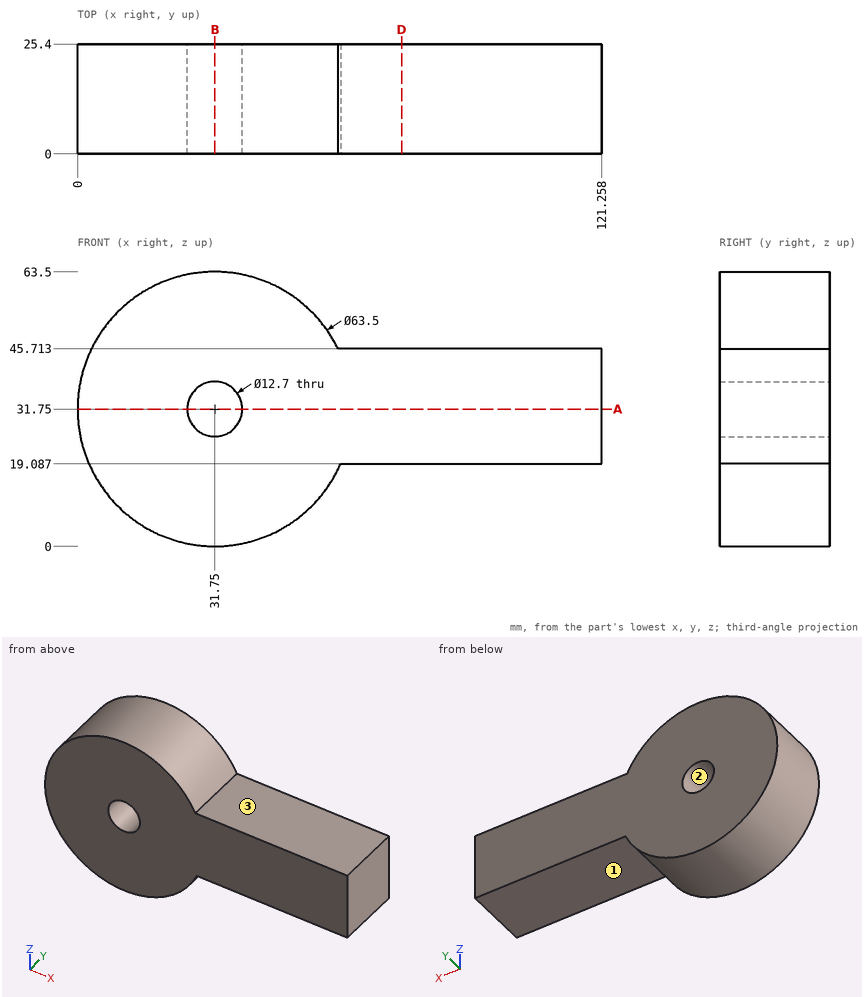
Could you check a few things on this drawing? It's one solid part, dimensions in mm from its lowest x, y, z. Coordinates: 2 decimals unless noted, no trailing zeros. Write each loop counter-clockwise with the first axis right and the second up, starting at its lowest first coordinate (ties: lowest second). Pieces come first, ordered by that corner, then holes. Notation, with made-up numbers: (46, 32) - (96, 32) arc R9 ccw to (96, 37) - close; hole circle Ø5 at (54.5, -36.5). An arc over 180 degrees is marked (long way). Put each result on its own line as item: value. Start each with the question number.
Q1. I want a section at A-A on z = 31.75. Write out the boundary of the cut face in (x, y), plus the area to 3 significant figures.
Q2. Please list where these lines run through material, in increasing order: L1, parallel to Z at x = 31.75, y = 14.5; L2, parallel to X at y = 20, z = 31.75; L3, parallel to Z at x = 112.5, y = 20.
Q3. I want a section at D-D on x = 75. Write out the boundary of the cut face in (y, z).
Q4. Thinking about a two-plate mould opening in Z: for the marked faces 1, 2 and 3, which applies, pulls with the +Z half, pulls with the -Z half, needs draft (parallel to the pull), parting line crosses it, or undercut?
Q5. I'm going to push flat-ended pins straight in: P1, Ø1, axis at y = 6.5, z = 15.5, coming from the +X side; P2, Ø1, axis at x = 35.5, y = 10, coming from the -Z side; P3, Ø5, axis at y = 3, z = 27.5, coming from the -X side; P4, Ø14.5, axis at x = 31.75, z = 31.75, coming from the -Y side. Where does each tip first touch, or does it pass through?
Q6. I want a section at B-B on x = 31.75. Write out the boundary of the cut face in (y, z).
Checks:
1. outline: (0, 0) - (25.4, 0) - (25.4, 25.4) - (0, 25.4) - close; (38.1, 0) - (121.26, 0) - (121.26, 25.4) - (38.1, 25.4) - close
1. area: 2,760 mm²
2. L1: 0 to 25.4, 38.1 to 63.5
2. L2: 0 to 25.4, 38.1 to 121.26
2. L3: 19.09 to 45.71
3. outline: (0, 19.09) - (25.4, 19.09) - (25.4, 45.71) - (0, 45.71) - close
4. face 1: pulls with the -Z half
4. face 2: undercut
4. face 3: pulls with the +Z half
5. P1: x = 59.32
5. P2: z = 0.17
5. P3: x = 0.05
5. P4: y = 0
6. outline: (0, 0) - (25.4, 0) - (25.4, 25.4) - (0, 25.4) - close; (0, 38.1) - (25.4, 38.1) - (25.4, 63.5) - (0, 63.5) - close
